Could you check a few things on this model? Use its own coordinates, in mm. A direction names the side the tool comes from. Give positions to 0.01 mm unless a question says otherwise; leave off trailing zeros. Order: outer loops, then holes, each group sorted by start corner. A loop starts at its lowest first (then second) coordinate and runs counter-clockwise, first axis right, second up. Notation, with made-up numbers: M -36.75,-38.75 L -6.75,-38.75 A28 cw -6.75,-14.75 Z; hole C 75.25,17 d2. An arc over 180 degrees is marked long. Use a Markdown table: item, result. Add a question column.
Item 1: Suppose I cut it at B-B on z = 27. Write out the boundary of the cut face in (x, y).
Item 2: If I drill on L1, parallel to Y at x = 32.5, z = 8; L2, parallel to X at y = -7.5, z = 15; L3, parallel to Y at x = 14, z = 19.5, over which ranges is the centre line in solid material (lowest first)? Write a range as from..to.
Item 3: Suppose I cut it at D-D on z = 3. Write out the boundary of the cut face in (x, y).
Item 4: I'm going to push flat-ended pins straight in: pin 1 Ø1 at (y, z) = (-29, 27.5) entering from -X; pin 2 Ø6 at (x, z) = (11.5, 16) entering from -Y; pin 3 Ø6 at (y, z) = (-27, 9) entering from -X; pin 4 Ø2 at (x, y) = (28.5, -13.5) entering from +Z. Where does each tip first touch, or does it pass through?
Item 5: Suppose I cut it at A-A on x = 34.5. Write out the boundary of the cut face in (y, z) (3 decimals).
Item 6: Suppose I cut it at C-C on x = 23.5. Write out the boundary of the cut face in (y, z) (3 decimals), plus the area to 3 significant figures.
Item 7: If we mould it in two halves opening along X, with no side actions, what happens to faces 1 (the face through (13.44, -18.85, 17.2)), 2 (the face through (24.73, -32.31, 17.38)), 3 (the face through (27.749, -6.994, 35.411)), 4 (the face through (34.175, -4.71, 23.55))? For each: released by +X, released by -X, zero draft, split by the parting line, or undercut.
Item 8: For faces 5 (the face through (15.831, -34.343, 31.894)), 6 (the face through (28.68, -5.72, 13.43)), 7 (the face through (25.4, -24, 21)), 8 (the face through (12.7, -9, 23)), 9 (the face through (29.096, -29.246, 27.577)), which set-ups out of +Z, -Z, +X, -X, +Y, -Y let a thin tool reach every point of the face, with its end or its side?
from build123d import *

# Parameters (mm, degrees)
F0_W     = 38.1
F0_H     = 38.1
F1_DEPTH = 38.1
F5_DEPTH = 38.1
F7_DEPTH = 38.1
F8_W     = 25.4
F8_H     = 7.62
F9_DEPTH = 38.1


with BuildPart() as f1:
    # F0 (on Front) → F1 (new body)
    with BuildSketch(Plane.XZ):
        with Locations((19.05, 19.05)):
            Rectangle(F0_W, F0_H)
    extrude(amount=F1_DEPTH)

    # F4 (on face) → F5 (cut)
    with BuildSketch(Plane.YZ.offset(38.1)):
        Polygon((-6.35, 38.1), (-31.75, 38.1), (-26.67, 16.755341), (-21.59, 28.575), (-16.51, 28.575), (-11.43, 16.885228), align=None)
        Polygon((-31.75, 0), (-38.1, 38.1), (-38.1, 0), align=None)
        Polygon((-19.05, 15.875), (-25.4, 0), (-12.7, 0), align=None)
        Polygon((0, 0), (0, 38.1), (-6.35, 0), align=None)
    extrude(amount=-F5_DEPTH, mode=Mode.SUBTRACT)

    # F6 (on offset) → F7 (cut)
    with BuildSketch(Plane.XZ.offset(38.1)):
        Polygon((0, 38.1), (0, 0), (6.35, 38.1), align=None)
        Polygon((25.4, 38.1), (12.7, 38.1), (19.05, 25.511248), align=None)
        Polygon((11.43, 22.225), (6.35, 0), (31.75, 0), (26.67, 22.225), (21.59, 9.525), (16.51, 9.525), align=None)
        Polygon((31.75, 38.1), (38.1, 0), (38.1, 38.1), align=None)
    extrude(amount=-F7_DEPTH, mode=Mode.SUBTRACT)

    # F8 (on offset) → F9 (cut)
    with BuildSketch(Plane.XY.offset(38.1)):
        with Locations((25.4, -11.43)):
            Rectangle(F8_W, F8_H)
        with Locations((12.7, -26.67)):
            Rectangle(F8_W, F8_H)
    extrude(amount=-F9_DEPTH, mode=Mode.SUBTRACT)


solid = f1.part
Findings below:
| question | item | result |
|---|---|---|
| 1 | outline | M 4.5,-36.25 L 18.3,-36.25 L 18.3,-30.48 L 4.5,-30.48 Z; M 4.5,-22.27 L 18.3,-22.27 L 18.3,-15.83 L 4.5,-15.83 Z; M 4.5,-9.01 L 12.7,-9.01 L 12.7,-7.62 L 18.3,-7.62 L 18.3,-1.85 L 4.5,-1.85 Z; M 19.8,-36.25 L 33.6,-36.25 L 33.6,-29.11 L 25.4,-29.11 L 25.4,-30.48 L 19.8,-30.48 Z; M 19.8,-22.27 L 33.6,-22.27 L 33.6,-15.83 L 19.8,-15.83 Z; M 19.8,-7.62 L 33.6,-7.62 L 33.6,-1.85 L 19.8,-1.85 Z |
| 2 | L1 | y = -33.08..-22.2, -15.9..-15.24, -7.62..-5.02 |
| 2 | L2 | x = 2.5..9.78, 14.32..23.78, 28.32..35.6 |
| 2 | L3 | y = -35..-30.48, -22.86..-15.24, -7.62..-3.1 |
| 3 | outline | M 0.5,-32.25 L 7.04,-32.25 L 7.04,-30.48 L 0.5,-30.48 Z; M 0.5,-13.9 L 7.04,-13.9 L 7.04,-5.85 L 0.5,-5.85 Z; M 31.06,-32.25 L 37.6,-32.25 L 37.6,-24.2 L 31.06,-24.2 Z; M 31.06,-7.62 L 37.6,-7.62 L 37.6,-5.85 L 31.06,-5.85 Z |
| 4 | pin 1 | stops at x = 25.4 |
| 4 | pin 2 | stops at y = -34.9 |
| 4 | pin 3 | stops at x = 29.01 |
| 4 | pin 4 | passes through |
| 5 | outline | M -35.35,21.6 L -31.75,0 L -25.4,0 L -19.05,15.875 L -15.24,6.35 L -15.24,21.6 L -24.588,21.6 L -26.67,16.755 L -27.823,21.6 Z; M -7.62,0 L -6.35,0 L -2.75,21.6 L -7.62,21.6 Z |
| 6 | outline | M -37.472,34.333 L -34.133,14.3 L -30.48,14.3 L -30.48,32.764 L -30.854,34.333 Z; M -22.86,14.3 L -19.68,14.3 L -19.05,15.875 L -18.42,14.3 L -15.24,14.3 L -15.24,25.653 L -16.51,28.575 L -21.59,28.575 L -22.86,25.62 Z; M -7.62,14.3 L -3.967,14.3 L -0.628,34.333 L -7.252,34.333 L -7.62,32.796 Z |
| 6 | area | 317 mm^2 |
| 7 | face 1 | undercut |
| 7 | face 2 | undercut |
| 7 | face 3 | zero draft |
| 7 | face 4 | released by +X |
| 8 | face 5 | +Z, +Y, -Y |
| 8 | face 6 | -Z, +Y, -Y |
| 8 | face 7 | +Z, -Z, -X |
| 8 | face 8 | +Z, -Z, +X |
| 8 | face 9 | +Z, +X, -X |
